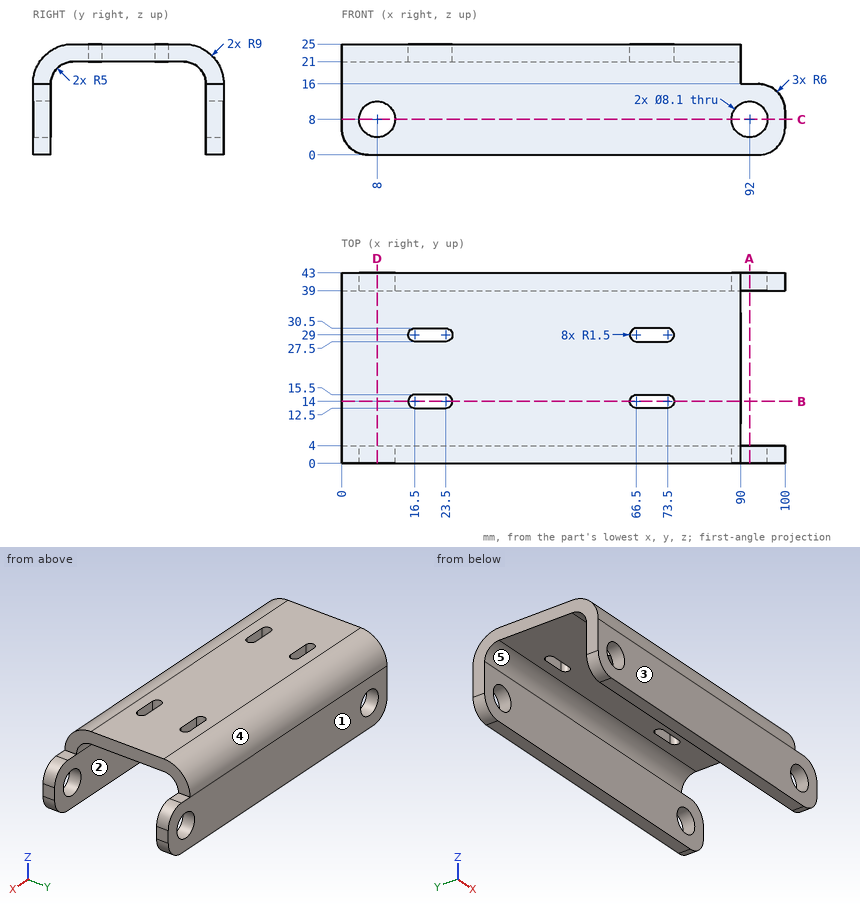
Could you check a few things on this drawing? It's one solid part, dimensions in mm from its lowest x, y, z. A direction names the side the tool comes from. Give positions to 0.01 mm unless a question says otherwise; leave off trailing zeros. Write each loop counter-clockwise with the first axis right and the second up, starting at its lowest first coordinate (ties: lowest second). Pieces come first, ordered by that corner, then holes. Notation, with made-up numbers: (64.25, 20.5) -> (80.25, 20.5) arc R26 cw to (80.25, 43.5) -> close; hole circle Ø3 at (-12, 34.5). An arc over 180 degrees is marked (long way). Answer as CSV lines item,"result". Start each with the question number.
(1) If we section it at A-A, the plane x = 92: Write out the boundary of the cut face in (y, z).
(2) If we section it at D-D, the plane x = 8: Write out the boundary of the cut face in (y, z).
(3) If we section it at C-C, the plane z = 8: Write out the boundary of the cut face in (x, y).
(4) I'm going to push flat-ended pins straight in: pin 1 Ø7.5 at (x, z) = (8, 8) entering from +Y; pin 2 Ø1.2 at (x, y) = (92.5, 1) entering from +Z; pin 3 Ø4 at (x, y) = (12, 38.5) entering from +Z; pin 4 Ø4.5 at (y, z) = (22, 20) entering from +X. Where does each tip first touch, or does it pass through?
(5) Please list where these lines run through material, in increasing order: line 1 (X direction, y = 40.75, z = 8); line 2 (Y direction, x = 56, z = 4.75); line 3 (Z direction, x = 62, y = 10.5).
(6) If we mould it in two halves opening along Y, with no side actions, what happens to the marked faces 1, 2 and 3? For each: +Y half, -Y half, draft (parallel to the pull), parting line (faces both ways), or undercut.
(7) If we section it at B-B, the plane y = 14: Write out the boundary of the cut face in (x, z), and give its area (3 significant figures).
(8) Which directions (+Z, -Z, +X, -X, +Y, -Y) give clear straight access to the entire face, cutting with the end or side of a thin tool? Please do the marked faces 4 and 5.
Answer list:
1,outline,"(0, 0) -> (4, 0) -> (4, 3.95) -> (0, 3.95) -> close; (0, 12.05) -> (4, 12.05) -> (4, 16) -> (0, 16) -> close; (39, 0) -> (43, 0) -> (43, 3.95) -> (39, 3.95) -> close; (39, 12.05) -> (43, 12.05) -> (43, 16) -> (39, 16) -> close"
2,outline,"(0, 0) -> (4, 0) -> (4, 3.95) -> (0, 3.95) -> close; (0, 12.05) -> (4, 12.05) -> (4, 16) arc R5 cw to (9, 21) -> (34, 21) arc R5 cw to (39, 16) -> (39, 12.05) -> (43, 12.05) -> (43, 16) arc R9 ccw to (34, 25) -> (9, 25) arc R9 ccw to (0, 16) -> close; (39, 0) -> (43, 0) -> (43, 3.95) -> (39, 3.95) -> close"
3,outline,"(0, 0) -> (3.95, 0) -> (3.95, 4) -> (0, 4) -> close; (0, 39) -> (3.95, 39) -> (3.95, 43) -> (0, 43) -> close; (12.05, 0) -> (87.95, 0) -> (87.95, 4) -> (12.05, 4) -> close; (12.05, 39) -> (87.95, 39) -> (87.95, 43) -> (12.05, 43) -> close; (96.05, 0) -> (100, 0) -> (100, 4) -> (96.05, 4) -> close; (96.05, 39) -> (100, 39) -> (100, 43) -> (96.05, 43) -> close"
4,pin 1,"through"
4,pin 2,"z = 16"
4,pin 3,"z = 24.65"
4,pin 4,"x = 90"
5,line 1,"0 to 3.95, 12.05 to 87.95, 96.05 to 100"
5,line 2,"0 to 4, 39 to 43"
5,line 3,"21 to 25"
6,face 1,"+Y half"
6,face 2,"undercut"
6,face 3,"-Y half"
7,outline,"(0, 21) -> (15, 21) -> (15, 25) -> (0, 25) -> close; (25, 21) -> (65, 21) -> (65, 25) -> (25, 25) -> close; (75, 21) -> (90, 21) -> (90, 25) -> (75, 25) -> close"
7,area,"280 mm^2"
8,face 4,"+Z, +X, -X, +Y"
8,face 5,"-Z, +X, -X"
